Design review of the part built by this model. Coordinates are the model's own, in mm. Coordinates: 2 decimals unless noted, no trailing zeros. Write each loop counter-clockwise with the first axis right and the second up, starting at its lowest first coordinate (ties: lowest second). Pieces come first, ordered by that corner, then holes.
Q1. Take a section at B-B, the plane y = -30. Write out the cut boundary in (x, z).
Q2. Take a section at D-D, the plane x = 38. Write out the cut boundary in (y, z).
Q3. For pin 1 Ø3.5 at (x, y) = (72.5, 35) entering from +Z, flat-tipped, find the tip position at first contact; note if it passes through.
Q4. For L1, parallel to Y at x = 72.5, z = 0.65; L2, parallel to X at y = 1, z = 1.5; L3, parallel to Y at x = 33.5, z = 1.5, list the stretches that pass through material, from the lowest coordinate up.
Q5. Take a section at C-C, the plane z = 1.6. State how many separate pieces and enclosed holes the cut face has, plus the area to 3 significant figures.
Q6. Take a section at A-A, the plane x = -72.5. Write out the cut boundary in (y, z), plus the area to 3 significant figures.
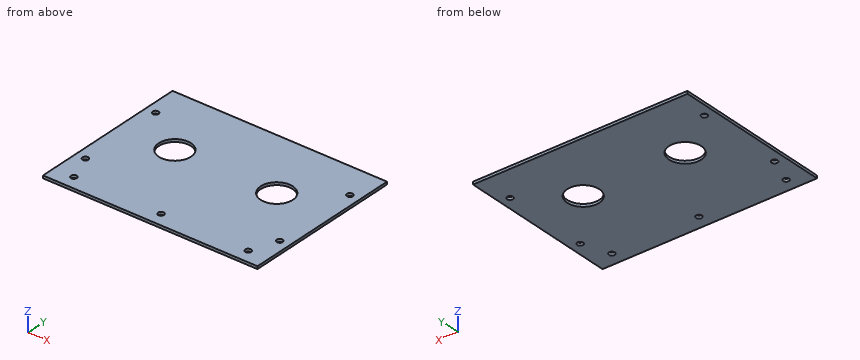
from build123d import *

# Parameters (mm, degrees)
SKETCH_1_W          = 160
SKETCH_1_H          = 120
EXTRUDE_1_DEPTH     = 2
SKETCH_2_R          = 2.2
SKETCH_2_R_2        = 12
CUT_EXTRUDE_1_DEPTH = 2
SKETCH_4_R          = 2.2
CUT_EXTRUDE_2_DEPTH = 105


with BuildPart() as part:
    # ｽｹｯﾁ1 → ﾎﾞｽ - 押し出し1 (new body)
    with BuildSketch(Plane.XY):
        Rectangle(SKETCH_1_W, SKETCH_1_H)
    extrude(amount=EXTRUDE_1_DEPTH)

    # ｽｹｯﾁ2 → ｶｯﾄ - 押し出し1 (cut)
    with BuildSketch(Plane.XY.offset(2)):
        with Locations((0, -50)):
            Circle(SKETCH_2_R)
        with Locations((-65, -50)):
            Circle(SKETCH_2_R)
        with Locations((-38, 10)):
            Circle(SKETCH_2_R_2)
        with Locations((38, 10)):
            Circle(SKETCH_2_R_2)
        with Locations((65, -50)):
            Circle(SKETCH_2_R)
    extrude(amount=-CUT_EXTRUDE_1_DEPTH, mode=Mode.SUBTRACT)

    # ｽｹｯﾁ4 → ｶｯﾄ - 押し出し2 (cut)
    with BuildSketch(Plane.XY.offset(2)):
        with Locations((72.5, 35)):
            Circle(SKETCH_4_R)
        with Locations((72.5, -30)):
            Circle(SKETCH_4_R)
        with Locations((-72.5, 35)):
            Circle(SKETCH_4_R)
        with Locations((-72.5, -30)):
            Circle(SKETCH_4_R)
    extrude(amount=-CUT_EXTRUDE_2_DEPTH, mode=Mode.SUBTRACT)


solid = part.part
Responses:
1. outline: (-80, 0) - (-74.7, 0) - (-74.7, 2) - (-80, 2) - close; (-70.3, 0) - (70.3, 0) - (70.3, 2) - (-70.3, 2) - close; (74.7, 0) - (80, 0) - (80, 2) - (74.7, 2) - close
2. outline: (-60, 0) - (-2, 0) - (-2, 2) - (-60, 2) - close; (22, 0) - (60, 0) - (60, 2) - (22, 2) - close
3. pin 1: passes through
4. L1: y = -60 to -32.2, -27.8 to 32.8, 37.2 to 60
4. L2: x = -80 to -45.94, -30.06 to 30.06, 45.94 to 80
4. L3: y = -60 to -1.12, 21.12 to 60
5. separate pieces: 1
5. enclosed holes: 9
5. area: 18,200 mm2
6. outline: (-60, 0) - (-32.2, 0) - (-32.2, 2) - (-60, 2) - close; (-27.8, 0) - (32.8, 0) - (32.8, 2) - (-27.8, 2) - close; (37.2, 0) - (60, 0) - (60, 2) - (37.2, 2) - close
6. area: 222 mm2
